Print and shaded views of the part. All mm, measured from the part's lowest x, y and z. Coordinates: 2 decimals unless noted, no trailing zeros. Write each loop counter-clockwise with the first axis right and the second up, starting at its lowest first coordinate (ties: lowest second). Pieces come first, ordered by that corner, then holes. Notation, with made-up numbers: (-18, 77.5) -> (15, 77.5) arc R24 ccw to (15, 99.5) -> close; hole circle Ø7 at (70.5, 56). An arc over 180 degrees is marked (long way). Write item = value, one per line.
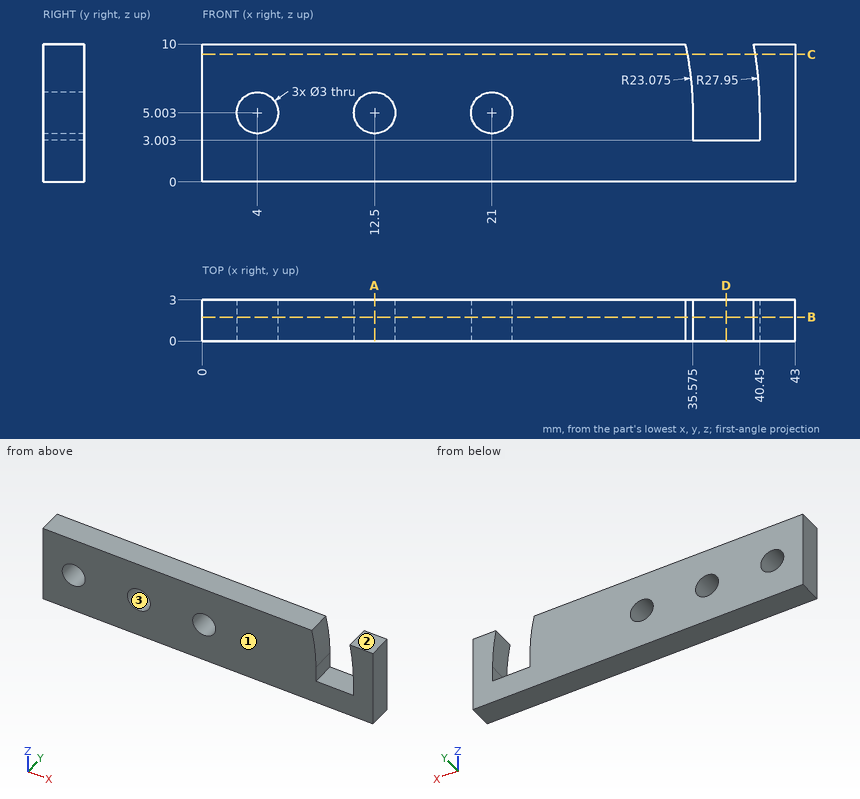
Q1. Saw through at B-B on y = 1.75. Count the separate pieces of the cut face and the enclosed holes in it.
Model answer:
separate_pieces = 1
enclosed_holes = 3
Q2. Saw through at A-A on x = 12.5. Give the cut face in (y, z), and give its area (3 significant figures).
Model answer:
outline = (0, 0) -> (3, 0) -> (3, 3.5) -> (0, 3.5) -> close; (0, 6.5) -> (3, 6.5) -> (3, 10) -> (0, 10) -> close
area = 21.0 mm²
Q3. Saw through at D-D on x = 38. Give the cut face in (y, z).
Model answer:
outline = (0, 0) -> (3, 0) -> (3, 3) -> (0, 3) -> close
Q4. Saw through at C-C on z = 9.25. Give the cut face in (x, y).
Model answer:
outline = (0, 0) -> (35.18, 0) -> (35.18, 3) -> (0, 3) -> close; (40.13, 0) -> (43, 0) -> (43, 3) -> (40.13, 3) -> close
Q5. Mould opens along Z. For the marked faces 1, 2 and 3 say: released by +Z, released by -Z, zero draft, split by the parting line, or undercut.
Model answer:
face_1 = zero draft
face_2 = released by +Z
face_3 = undercut
Q6. Pin check, flat tip, straight feed: pin 1 (0.9 mm diameter, centred on x = 39, y = 2, fed in from +Z). Stop position of the tip, or through.
Model answer:
pin_1 = 3
Q7. Probe line 1 (Z direction, x = 21, y = 2.05); line 2 (Z direction, x = 38.5, y = 1.2); line 3 (X direction, y = 2.4, z = 5.5) (1 decimal). List the from-to ranges inside material, lowest first. Write a range as from..to.
Model answer:
line_1 = 0..3.5, 6.5..10
line_2 = 0..3
line_3 = 0..2.6, 5.4..11.1, 13.9..19.6, 22.4..35.6, 40.4..43
